```python
from build123d import *

# Parameters (mm, degrees)
SKETCH1_W           = 55
SKETCH1_H           = 71
BOSS_EXTRUDE1_DEPTH = 20
CUT_EXTRUDE1_DEPTH  = 20


with BuildPart() as part:
    # Sketch1 → Boss-Extrude1 (new body)
    with BuildSketch(Plane(origin=(0, 0, 0), x_dir=(1, 0, 0), z_dir=(0, 1, 0))):
        with BuildLine():
            Line((29.5, -35.5), (29.5, 35.5))
            ThreePointArc((29.5, 35.5), (28.914213562, 36.914213562), (27.5, 37.5))
            Line((27.5, 37.5), (-27.5, 37.5))
            ThreePointArc((-27.5, 37.5), (-28.914213562, 36.914213562), (-29.5, 35.5))
            Line((-29.5, 35.5), (-29.5, -35.5))
            ThreePointArc((-29.5, -35.5), (-28.914213562, -36.914213562), (-27.5, -37.5))
            Line((-27.5, -37.5), (27.5, -37.5))
            ThreePointArc((27.5, -37.5), (28.914213562, -36.914213562), (29.5, -35.5))
        make_face()
        Rectangle(SKETCH1_W, SKETCH1_H, mode=Mode.SUBTRACT)
    extrude(amount=BOSS_EXTRUDE1_DEPTH)

    # Sketch2 → Cut-Extrude1 (cut)
    with BuildSketch(Plane.ZY.offset(29.5)):
        with BuildLine():
            Line((-24.5, 15), (29.5, 15))
            ThreePointArc((29.5, 15), (31.621320344, 14.121320344), (32.5, 12))
            Line((32.5, 12), (32.5, -3))
            Line((32.5, -3), (-27.5, -3))
            Line((-27.5, -3), (-27.5, 12))
            ThreePointArc((-27.5, 12), (-26.621320344, 14.121320344), (-24.5, 15))
        make_face()
    extrude(amount=-CUT_EXTRUDE1_DEPTH, mode=Mode.SUBTRACT)


solid = part.part
```
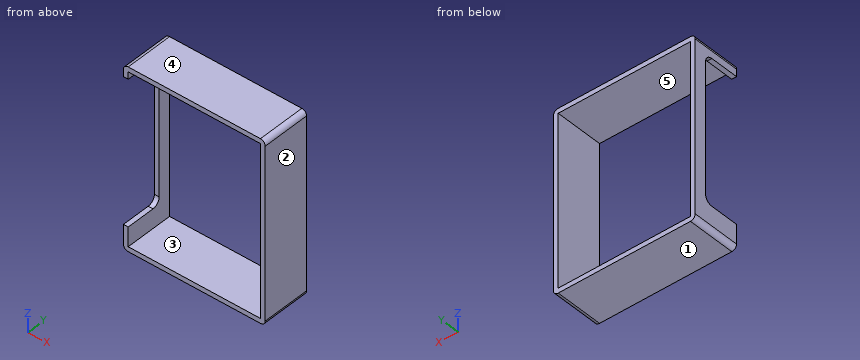
Design review of the part built by this model. Coordinates are the model's own, in mm. Face numbers are marked on the shaded views. A direction names the side the tool comes from. Give positions to 0.01 mm unless a question says otherwise; leave off trailing zeros. Loops run counter-clockwise (first coordinate to the right, second up) from the corner with the lowest first, then second, coordinate; pieces in that order, holes last. Notation, with made-up numbers: (77.25, 26.25) -> (81.25, 26.25) arc R31 cw to (81.25, 61.25) -> close; hole circle Ø5 at (1, 2). An arc over 180 degrees is marked (long way). Write each question's results on one line, items separated by ' | '.
Q1. Take a section at D-D, the plane y = 13. Write out the cut boundary in (x, z), plus the area to 3 significant figures.
Reply:
outline: (-29.5, -35.5) arc R2 ccw to (-27.5, -37.5) -> (27.5, -37.5) arc R2 ccw to (29.5, -35.5) -> (29.5, 35.5) arc R2 ccw to (27.5, 37.5) -> (-27.5, 37.5) arc R2 ccw to (-29.5, 35.5) -> (-29.5, 32.33) -> (-27.5, 32.33) -> (-27.5, 35.5) -> (27.5, 35.5) -> (27.5, -35.5) -> (-27.5, -35.5) -> (-27.5, -27.33) -> (-29.5, -27.33) -> close | area: 397 mm²
Q2. Take a section at B-B, the plane z = -30.5. Write out the cut boundary in (x, y).
Reply:
outline: (-29.5, 0) -> (-27.5, 0) -> (-27.5, 20) -> (-29.5, 20) -> close; (27.5, 0) -> (29.5, 0) -> (29.5, 20) -> (27.5, 20) -> close
Q3. Take a section at A-A, the plane x = 5. Write out the cut boundary in (y, z).
Reply:
outline: (0, -37.5) -> (20, -37.5) -> (20, -35.5) -> (0, -35.5) -> close; (0, 35.5) -> (20, 35.5) -> (20, 37.5) -> (0, 37.5) -> close
Q4. Wall thickness on L1, parallel to Z at x = -15.5, y = 5; L2, parallel to X at y = 4, z = -33.5; L3, parallel to X at y = 12.5, z = 1.5: over which ranges is each line inside the solid? List them lowest first.
Reply:
L1: z = -37.5 to -35.5, 35.5 to 37.5 | L2: x = -29.5 to -27.5, 27.5 to 29.5 | L3: x = 27.5 to 29.5
Q5. Machinability: for the marked faces 4 and 5, which of the approach directions +Z, -Z, +X, -X, +Y, -Y give a long, thin tool a straight path to every point of the face, cutting with its end or side? Answer none if there is none.
Reply:
face 4: +Z, +X, -X, +Y, -Y | face 5: +Y, -Y
Q6. The part is to be moulded in two halves that separate along X. For the marked faces 1, 2 and 3, say which applies: +X half, -X half, draft (parallel to the pull), parting line (faces both ways), or undercut.
Reply:
face 1: draft | face 2: +X half | face 3: undercut
Q7. For pin 1 Ø5 at (y, z) = (5, 16.5) entering from -X; pin 2 Ø1 at (x, y) = (-29, 5) entering from -Z; pin 3 Ø1.6 at (x, y) = (-29, 7) entering from +Z, all flat-tipped, find the tip position at first contact; note any pin that passes through.
Reply:
pin 1: stops at x = 27.5 | pin 2: stops at z = -37.23 | pin 3: stops at z = 37.37
Q8. Take a section at C-C, the plane y = 4.25. Write out the cut boundary in (x, z).
Reply:
outline: (-29.5, -35.5) arc R2 ccw to (-27.5, -37.5) -> (27.5, -37.5) arc R2 ccw to (29.5, -35.5) -> (29.5, 35.5) arc R2 ccw to (27.5, 37.5) -> (-27.5, 37.5) arc R2 ccw to (-29.5, 35.5) -> (-29.5, 32.5) -> (-27.5, 32.5) -> (-27.5, 35.5) -> (27.5, 35.5) -> (27.5, -35.5) -> (-27.5, -35.5) -> (-27.5, -27.5) -> (-29.5, -27.5) -> close
